from build123d import *

# Parameters (mm, degrees)
SKETCH1_R           = 0.81
BOSS_EXTRUDE1_DEPTH = 3


with BuildPart() as part:
    # Sketch1 → Boss-Extrude1 (new body)
    with BuildSketch(Plane(origin=(0, 0, 0), x_dir=(1, 0, 0), z_dir=(0, 1, 0))):
        Polygon((5.6453129, 2.562826463), (6.3943589, 2.877662463), (6.8624159, 2.950894463), (8.3003709, 2.699622463), (8.4974959, 1.934301463), (7.3598559, 1.019628463), (6.9146609, 0.857633463), (6.1067249, 0.771435463), (6.0924239, -0.702085537), (6.8985319, -0.803957537), (7.3404979, -0.974570537), (8.4601699, -1.911153537), (8.2482219, -2.672493537), (6.8056559, -2.895801537), (6.3391139, -2.813510537), (5.5963139, -2.484188537), (4.8471689, -3.753135537), (5.4943549, -4.244415537), (5.7917899, -4.613151537), (6.2931629, -5.984095537), (5.7289469, -6.537468537), (4.3679989, -6.009575537), (4.0051049, -5.705026537), (3.5264829, -5.048435537), (2.2432229, -5.772805537), (2.5580589, -6.521851537), (2.6312909, -6.989908537), (2.3800189, -8.427863537), (1.6146979, -8.624988537), (0.7000259, -7.487348537), (0.5380299, -7.042153537), (0.4518319, -6.234217537), (-1.0216891, -6.219916537), (-1.1235611, -7.026024537), (-1.2941741, -7.467990537), (-2.2307561, -8.587662537), (-2.9920971, -8.375714537), (-3.2154051, -6.933148537), (-3.1331131, -6.466606537), (-2.8037921, -5.723806537), (-4.0727391, -4.974661537), (-4.5640191, -5.621847537), (-4.9327541, -5.919282537), (-6.3036991, -6.420655537), (-6.8570721, -5.856439537), (-6.3291791, -4.495491537), (-6.0246291, -4.132597537), (-5.3680391, -3.653975537), (-6.0924091, -2.370715537), (-6.8414551, -2.685551537), (-7.3095121, -2.758783537), (-8.7474671, -2.507511537), (-8.9445921, -1.742190537), (-7.8069511, -0.827518537), (-7.3617561, -0.665522537), (-6.5538201, -0.579324537), (-6.5395191, 0.894196463), (-7.3456281, 0.996068463), (-7.7875941, 1.166681463), (-8.9072661, 2.103264463), (-8.6953181, 2.864604463), (-7.2527521, 3.087912463), (-6.7862101, 3.005620463), (-6.0434091, 2.676299463), (-5.2942651, 3.945246463), (-5.9414511, 4.436526463), (-6.2388861, 4.805262463), (-6.7402581, 6.176206463), (-6.1760431, 6.729579463), (-4.8150951, 6.201686463), (-4.4522011, 5.897137463), (-3.9735791, 5.240546463), (-2.6903191, 5.964916463), (-3.0051541, 6.713962463), (-3.0783871, 7.182019463), (-2.8271151, 8.619974463), (-2.0617941, 8.817099463), (-1.1471211, 7.679458463), (-0.9851261, 7.234264463), (-0.8989281, 6.426327463), (0.5745929, 6.412026463), (0.6764649, 7.218135463), (0.8470779, 7.660101463), (1.7836609, 8.779773463), (2.5450009, 8.567825463), (2.7683089, 7.125259463), (2.6860179, 6.658717463), (2.3566959, 5.915916463), (3.6256429, 5.166772463), (4.1169229, 5.813958463), (4.4856589, 6.111393463), (5.8566029, 6.612765463), (6.4099759, 6.048550463), (5.8820829, 4.687602463), (5.5775339, 4.324708463), (4.9209439, 3.846086463), align=None)
        with Locations(Location((-0.2235476, 0.096055463, 0), (0, 0, 270))):
            Circle(SKETCH1_R, mode=Mode.SUBTRACT)
    extrude(amount=BOSS_EXTRUDE1_DEPTH)


solid = part.part
CAD build for the part. Positions are in the model's coordinates, mm. A direction names the side the tool comes from. Give positions to 0.01 mm unless a question says otherwise; leave off trailing zeros. Loops run counter-clockwise (first coordinate to the right, second up) from the corner with the lowest first, then second, coordinate; pieces in that order, holes last. Notation, with made-up numbers: M -11,73 L 23,73 A28 ccw 23,110 Z; hole C 34,13.5 d4. An arc over 180 degrees is marked long. Answer in a Markdown table with one row per item. Add a question column.
Item 1: Band-saw the part on B-B on z = -1.5. Give the cut face in (x, y), then the cut area to 3 significant figures.
Item 2: Band-saw the part on A-A on z = -5.5. Give the cut face in (x, y), then the cut area to 3 significant figures.
Item 3: Probe probe 1 along Z at (x, y) = (-0.5, 1); probe 2 along X at (y, z) = (0.75, -7); probe 3 along X at (y, z) = (0.65, 5.5). List the from-to ranges inside material, lowest first.
Item 4: Tool access for faces 5 (the face through (-1.756, 1.479, 8.02)), 6 (the face through (-0.943, 1.479, -6.836)), 7 (the face through (-8.38, 1.48, 1.29)): list every direction of +Z, -Z, +X, -X, +Y, -Y with a clear straight run to the whole face (end or side of a thin tool).
Item 5: Band-saw the part on C-C on z = 3.25. Give the cut face in (x, y).
Item 6: Drop flat-ended pins along their axis: P1, Ø1, axis at y = 2.5, z = -7, coming from the -X side; P2, Ø1.5, axis at x = 1, y = 2, coming from the -Z side. Give the stop position or say it passes through.
Item 7: Mould opens along Z. For faces 1 (the face through (7.892, 1.479, 1.436)), 2 (the face through (-2, 0, 0)), 3 (the face through (5.28, 1.48, -3.21)), 4 (the face through (-5.609, 1.479, 6.166)) say: +Z half, -Z half, draft (parallel to the pull), parting line (faces both ways), or undercut.
Reply:
| question | item | result |
|---|---|---|
| 1 | outline | M -8.19,0 L 7.96,0 L 7.96,3 L -8.19,3 Z |
| 1 | area | 48.4 mm^2 |
| 2 | outline | M -6.49,0 L -4.16,0 L -4.16,3 L -6.49,3 Z; M -3.51,0 L 3.06,0 L 3.06,3 L -3.51,3 Z; M 3.88,0 L 6.2,0 L 6.2,3 L 3.88,3 Z |
| 2 | area | 33.7 mm^2 |
| 3 | probe 1 | z = -6.42 to -0.86, 0.67 to 6.22 |
| 3 | probe 2 | x = -3.05 to -0.96, 0.65 to 2.75 |
| 3 | probe 3 | x = -6.72 to -4.47, -3.18 to 2.73, 3.86 to 6.12 |
| 4 | face 5 | +Z, +Y, -Y |
| 4 | face 6 | -Z, +Y, -Y |
| 4 | face 7 | -X, +Y, -Y |
| 5 | outline | M -5.6,0 L 5.14,0 L 5.14,3 L -5.6,3 Z |
| 6 | P1 | stops at x = -6.41 |
| 6 | P2 | stops at z = -8.74 |
| 7 | face 1 | undercut |
| 7 | face 2 | draft |
| 7 | face 3 | undercut |
| 7 | face 4 | +Z half |
